For this review, take the finished solid that the model builds, in its own axes (mm). Face numbers are marked on the shaded views. A direction names the side the tool comes from. Coordinates: 2 decimals unless noted, no trailing zeros. Loops run counter-clockwise (first coordinate to the right, second up) from the corner with the lowest first, then second, coordinate; pieces in that order, holes last. Notation, with made-up numbers: (-8, -25.5) -> (8, -25.5) arc R34 cw to (8, 7.5) -> close; hole circle Ø10 at (75.25, 68). An arc over 180 degrees is marked (long way). One line per item, written item: value.
from build123d import *

# Parameters (mm, degrees)
CROQUIS1_W             = 19
CROQUIS1_H             = 10
BRIDA_BASE1_DEPTH      = 2
BRIDA_DE_ARISTA1_DEPTH = 15
CORTAR_EXTRUIR1_REACH  = 62.77
REDONDEO1_R            = 1


# Sheet-metal steps are written as plain solids
with BuildPart() as part:
    # Croquis1 → Brida base1 (new body)
    with BuildSketch(Plane.XY):
        with Locations((9.5, -5)):
            Rectangle(CROQUIS1_W, CROQUIS1_H)
        with BuildLine():
            Line((5.25, -4.5), (5.25, -5.5))
            ThreePointArc((5.25, -5.5), (3.5, -7.25), (1.75, -5.5))
            Line((1.75, -5.5), (1.75, -4.5))
            ThreePointArc((1.75, -4.5), (3.5, -2.75), (5.25, -4.5))
        make_face(mode=Mode.SUBTRACT)
        with BuildLine():
            Line((17.25, -4.5), (17.25, -5.5))
            ThreePointArc((17.25, -5.5), (15.5, -7.25), (13.75, -5.5))
            Line((13.75, -5.5), (13.75, -4.5))
            ThreePointArc((13.75, -4.5), (15.5, -2.75), (17.25, -4.5))
        make_face(mode=Mode.SUBTRACT)
    extrude(amount=-BRIDA_BASE1_DEPTH)

    # Brida de arista1 section (across the edge) → Brida de arista1 (add)
    with BuildSketch(Plane(origin=(17, 2, 0), x_dir=(0, -1, 0), z_dir=(-1, 0, 0))):
        with BuildLine():
            Line((-2, 2), (-2, 56))
            Line((-2, 56), (0, 56))
            Line((0, 56), (0, 2))
            ThreePointArc((0, 2), (0.585786438, 0.585786438), (2, 0))
            Line((2, 0), (2, -2))
            ThreePointArc((2, -2), (-0.828427125, -0.828427125), (-2, 2))
        make_face()
    extrude(amount=BRIDA_DE_ARISTA1_DEPTH)

    # Croquis9 → Cortar-Extruir1 (cut, up to next)
    with BuildSketch(Plane(origin=(0, 4, 0), x_dir=(1, 0, 0), z_dir=(0, 1, 0)), mode=Mode.PRIVATE) as cortar_extruir1_sk1:
        with BuildLine():
            Line((7.75, -11), (7.75, -5))
            ThreePointArc((7.75, -5), (9.5, -3.25), (11.25, -5))
            Line((11.25, -5), (11.25, -11))
            ThreePointArc((11.25, -11), (9.5, -12.75), (7.75, -11))
        make_face()
    cortar_extruir1_tool1 = extrude(cortar_extruir1_sk1.sketch, amount=-CORTAR_EXTRUIR1_REACH, mode=Mode.PRIVATE) & part.part
    # Croquis9 → Cortar-Extruir1 (cut, up to next)
    with BuildSketch(Plane(origin=(0, 4, 0), x_dir=(1, 0, 0), z_dir=(0, 1, 0)), mode=Mode.PRIVATE) as cortar_extruir1_sk2:
        with BuildLine():
            Line((7.75, -51), (7.75, -45))
            ThreePointArc((7.75, -45), (9.5, -43.25), (11.25, -45))
            Line((11.25, -45), (11.25, -51))
            ThreePointArc((11.25, -51), (9.5, -52.75), (7.75, -51))
        make_face()
    cortar_extruir1_tool2 = extrude(cortar_extruir1_sk2.sketch, amount=-CORTAR_EXTRUIR1_REACH, mode=Mode.PRIVATE) & part.part
    add(cortar_extruir1_tool1.solids().sort_by_distance((9.5, 4, 8))[0], mode=Mode.SUBTRACT)
    add(cortar_extruir1_tool2.solids().sort_by_distance((9.5, 4, 48))[0], mode=Mode.SUBTRACT)

    # Redondeo1
    redondeo1_edges = [part.edges().sort_by_distance(p)[0] for p in [
        (17, 3, 56),
        (2, 3, 56),
        (0, 0, -1),
        (19, 0, -1),
        (19, -10, -1),
        (0, -10, -1),
    ]]
    fillet(redondeo1_edges, radius=REDONDEO1_R)


solid = part.part
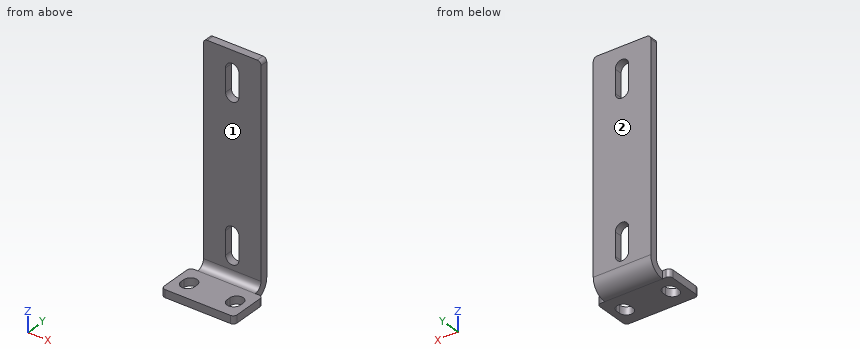
1. For the marked faces 1 and 2, list the 3-axis set-ups (+Z, -Z, +X, -X, +Y, -Y) from which the entire face can be reached by the end or side of a thin tool; tool diameter is ignored.
Return value:
face 1: +Z, +X, -X, -Y
face 2: +Z, -Z, +X, -X, +Y
2. Take a section at A-A, the plane z = 8.5. Give the boundary of the cut face in (x, y), and give its area (3 significant figures).
Return value:
outline: (2, 2) -> (7.75, 2) -> (7.75, 4) -> (2, 4) -> close; (11.25, 2) -> (17, 2) -> (17, 4) -> (11.25, 4) -> close
area: 23.0 mm2
3. Take a section at B-B, the plane x = 14.5. Give the boundary of the cut face in (y, z).
Return value:
outline: (-10, -2) -> (-6.94, -2) -> (-6.94, 0) -> (-10, 0) -> close; (-3.06, -2) -> (0, -2) arc R4 ccw to (4, 2) -> (4, 56) -> (2, 56) -> (2, 2) arc R2 cw to (0, 0) -> (-3.06, 0) -> close
4. To check wall thickness, follow probe 1 along Z at (x, y) = (9.75, 2.5); probe 2 along Z at (x, y) = (5.75, -2); probe 3 along Y at (x, z) = (14.5, 18.5). State the ranges of each line that lie inside material, in increasing order. Write a range as from..to.
Return value:
probe 1: z = -1.12..3.27, 12.73..43.27, 52.73..56
probe 2: z = -2..0
probe 3: y = 2..4
5. Take a section at D-D, the plane y = 2.75. Give the boundary of the cut face in (x, z), and give its area (3 significant figures).
Return value:
outline: (2, -0.9) -> (17, -0.9) -> (17, 55) arc R1 ccw to (16, 56) -> (3, 56) arc R1 ccw to (2, 55) -> close; hole (7.75, 5) arc R1.75 ccw to (11.25, 5) -> (11.25, 11) arc R1.75 ccw to (7.75, 11) -> close; hole (7.75, 45) arc R1.75 ccw to (11.25, 45) -> (11.25, 51) arc R1.75 ccw to (7.75, 51) -> close
area: 792 mm2
6. Take a section at C-C, the plane x = 9.5. Give the boundary of the cut face in (y, z), and give its area (3 significant figures).
Return value:
outline: (-10, -2) -> (0, -2) arc R4 ccw to (4, 2) -> (4, 3.25) -> (2, 3.25) -> (2, 2) arc R2 cw to (0, 0) -> (-10, 0) -> close; (2, 12.75) -> (4, 12.75) -> (4, 43.25) -> (2, 43.25) -> close; (2, 52.75) -> (4, 52.75) -> (4, 56) -> (2, 56) -> close
area: 99.4 mm2
7. Insertion check: pin 1 Ø3 at (y, z) = (2.5, 19.5) entering from +X; pin 2 Ø1.6 at (y, z) = (2.5, 8.5) entering from -X; pin 3 Ø6 at (x, y) = (9.5, -8.5) entering from +Z. Each pin has a flat end and moves straight along its axis. Give the tip position at first contact, or say it passes through.
Return value:
pin 1: stops at x = 17
pin 2: stops at x = 2
pin 3: stops at z = 0
